The listing builds one solid part. Answer for the finished solid, in the listing's coordinates (mm). Round coordinates to 2 decimals unless told otherwise and drop trailing zeros. Loops run counter-clockwise (first coordinate to the right, second up) from the corner with the lowest first, then second, coordinate; pieces in that order, holes last. Notation, with made-up numbers: (21.5, -24) -> (55.5, -24) arc R13 ccw to (55.5, -3) -> close; hole circle Ø2 at (-19.75, -18). An arc over 180 degrees is marked (long way). Use a Markdown table: item, result. Add a question column.
Q1. Section A-A on y = -0.95 is taken. Give the vertices of the cut face in (x, z).
Q2. Consider line 1 (X direction, y = -1.5, z = -0.5); line 2 (X direction, y = -0.8, z = -1.5); line 3 (Z direction, x = -38, y = -1.9). Determine where each line is inside the solid, lowest interval first.
Q3. Section B-B on x = 0 is taken. Give the vertices of the cut face in (y, z).
from build123d import *

# Parameters (mm, degrees)
F0_W     = 85
F0_H     = 9
F0_R     = 1.5
F1_DEPTH = 2
F2_R     = 4
F3_SIZE  = 1.87


with BuildPart() as f1:
    # F0 (on Front) → F1 (new body)
    with BuildSketch(Plane.XZ):
        Rectangle(F0_W, F0_H)
        with Locations((-38, 0)):
            Circle(F0_R, mode=Mode.SUBTRACT)
        Circle(F0_R, mode=Mode.SUBTRACT)
        with Locations((38, 0)):
            Circle(F0_R, mode=Mode.SUBTRACT)
    extrude(amount=F1_DEPTH)

    # F2
    f2_edges = [f1.edges().sort_by_distance(p)[0] for p in [
        (-42.5, -1, 4.5),
        (-42.5, -1, -4.5),
        (42.5, -1, -4.5),
        (42.5, -1, 4.5),
    ]]
    fillet(f2_edges, radius=F2_R)

    # F3
    f3_edges = [f1.edges().sort_by_distance(p)[0] for p in [
        (36.5, -2, 0),
        (-1.5, -2, 0),
        (-39.5, 0, 0),
    ]]
    chamfer(f3_edges, length=F3_SIZE)


solid = f1.part
Checked values:
| question | item | result |
|---|---|---|
| 1 | outline | (-42.5, -0.5) arc R4 ccw to (-38.5, -4.5) -> (38.5, -4.5) arc R4 ccw to (42.5, -0.5) -> (42.5, 0.5) arc R4 ccw to (38.5, 4.5) -> (-38.5, 4.5) arc R4 ccw to (-42.5, 0.5) -> close; hole circle Ø4.84 at (-38, 0); hole circle Ø4.64 at (0, 0); hole circle Ø4.64 at (38, 0) |
| 2 | line 1 | x = -42.5 to -39.8, -36.2 to -2.83, 2.83 to 35.17, 40.83 to 42.5 |
| 2 | line 2 | x = -42.37 to -40.09, -35.91 to -1.57, 1.57 to 36.43, 39.57 to 42.37 |
| 2 | line 3 | z = -4.5 to -1.5, 1.5 to 4.5 |
| 3 | outline | (-2, -4.5) -> (0, -4.5) -> (0, -1.5) -> (-0.13, -1.5) -> (-2, -3.37) -> close; (-2, 3.37) -> (-0.13, 1.5) -> (0, 1.5) -> (0, 4.5) -> (-2, 4.5) -> close |
